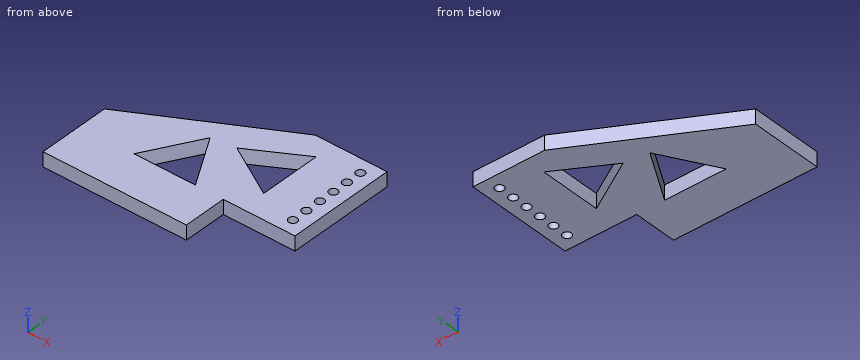
```python
from build123d import *

# Parameters (mm, degrees)
PAD_DEPTH           = 2
SKETCH001_R         = 0.6
HOLE_DEPTH          = 2.001
LINEARPATTERN_COUNT = 6
LINEARPATTERN_PITCH = 2.2
POCKET_DEPTH        = 2.001


with BuildPart() as part:
    # Sketch → Pad (new body)
    with BuildSketch(Plane.XY):
        Polygon((0, 0), (20, 0), (20, 6), (30, 6), (30, 21), (20, 21), (0, 10), align=None)
    extrude(amount=PAD_DEPTH)

    # Sketch001 (on Face9 of Pad) → Hole (cut, through all)
    with BuildSketch(Plane.XY.offset(2)):
        with Locations((28, 19)):
            Circle(SKETCH001_R)
    hole = extrude(amount=-HOLE_DEPTH, mode=Mode.SUBTRACT)

    # LinearPattern: Hole ×6
    with Locations(*[(0, -i * LINEARPATTERN_PITCH, 0) for i in range(1, LINEARPATTERN_COUNT)]):
        add(hole, mode=Mode.SUBTRACT)

    # Sketch002 (on Face5 of LinearPattern) → Pocket (cut, through all)
    with BuildSketch(Plane.XY.offset(2)):
        Polygon((11.837454, 13.403028), (7.563314, 6), (16.111595, 6), align=None)
        Polygon((22.577143, 9.579128), (22.577143, 18.127408), (15.174115, 13.853268), align=None)
    extrude(amount=-POCKET_DEPTH, mode=Mode.SUBTRACT)


solid = part.part
```
Check sheet for the modelled part. Datum: model origin and axes. Units: mm. Give positions to 0.01 mm unless a question says otherwise; leave off trailing zeros. Order: outer loops, then holes, each group sorted by start corner. A loop starts at its lowest first (then second) coordinate and runs counter-clockwise, first axis right, second up. Notation, with made-up numbers: (56.25, 57) -> (113.25, 57) arc R16 ccw to (113.25, 77) -> close; hole circle Ø2 at (80.5, -12.75). An arc over 180 degrees is marked (long way). Return JSON: item names as keys, results as strings.
1. Cross-section at B-B, the plane z = 0.75. Count the separate pieces of the cut face and the enclosed holes in it, plus the area to 3 significant figures.
From the geometry:
{"separate pieces": "1", "enclosed holes": "8", "area": "390 mm^2"}
2. Cross-section at D-D, the plane x = 13. Record the cut outline in (y, z).
From the geometry:
{"outline": "(0, 0) -> (6, 0) -> (6, 2) -> (0, 2) -> close; (11.39, 0) -> (17.15, 0) -> (17.15, 2) -> (11.39, 2) -> close"}
3. Cross-section at C-C, the plane x = 28. Record the cut outline in (y, z), plus the area to 3 significant figures.
From the geometry:
{"outline": "(6, 0) -> (7.4, 0) -> (7.4, 2) -> (6, 2) -> close; (8.6, 0) -> (9.6, 0) -> (9.6, 2) -> (8.6, 2) -> close; (10.8, 0) -> (11.8, 0) -> (11.8, 2) -> (10.8, 2) -> close; (13, 0) -> (14, 0) -> (14, 2) -> (13, 2) -> close; (15.2, 0) -> (16.2, 0) -> (16.2, 2) -> (15.2, 2) -> close; (17.4, 0) -> (18.4, 0) -> (18.4, 2) -> (17.4, 2) -> close; (19.6, 0) -> (21, 0) -> (21, 2) -> (19.6, 2) -> close", "area": "15.6 mm^2"}
4. Material ranges on probe 1 along X at (y, z) = (8.25, 0.3); probe 2 along Y at (x, z) = (9, 1); probe 3 along X at (y, z) = (4.25, 0.45), recorded low to high. Write a range as [from, to].
From the geometry:
{"probe 1": "[0, 8.86], [14.81, 27.45], [28.55, 30]", "probe 2": "[0, 6], [8.49, 14.95]", "probe 3": "[0, 20]"}
5. Cross-section at A-A, the plane y = 12.4. Record the cut outline in (x, z), plus the area to 3 significant figures.
From the geometry:
{"outline": "(4.36, 0) -> (11.26, 0) -> (11.26, 2) -> (4.36, 2) -> close; (12.42, 0) -> (17.69, 0) -> (17.69, 2) -> (12.42, 2) -> close; (22.58, 0) -> (27.4, 0) -> (27.4, 2) -> (22.58, 2) -> close; (28.6, 0) -> (30, 0) -> (30, 2) -> (28.6, 2) -> close", "area": "36.8 mm^2"}
6. Go/stop test with flat-tipped pins: P1, Ø0.6, axis at y = 12, z = 1, coming from the -X side; P2, Ø1, axis at x = 27, z = 1.5, coming from the -Y side; P3, Ø0.6, axis at x = 13, z = 0.5, coming from the +Y side (3 decimals). Record where each tip stops, or that it passes through.
From the geometry:
{"P1": "x = 3.09", "P2": "y = 6", "P3": "y = 17.315"}
